Input: part model. Units: mm. Frame: model coordinates. A direction names the side the tool comes from. Round coordinates to 2 decimals unless told otherwise and drop trailing zeros. Loops run counter-clockwise (first coordinate to the right, second up) from the corner with the lowest first, then second, coordinate; pieces in that order, holes last.
(1) Line query: line 1 (Y direction, x = 10.5, z = -10.5); line 2 (Z direction, x = 7.5, y = 22); line 3 (Z direction, x = 9.75, y = 4.5). Output: solid intervals per line, ascending.
(2) Cut plane C-C, the plane x = 12.5. Output: boundary loops of the cut face in (y, z), and give its area (3 significant figures).
(3) Access query for faces 4 (the face through (15, 10, 0)), 5 (the face through (12, 2.8, 12)), 6 (the face through (0, 28, 13.5)), 7 (the face through (-3, 14, 13.5)). Directions: +Z, -Z, +X, -X, +Y, -Y. A direction counts if a zero-diameter tool reaches every point of the face in a straight line with its end or side. Return the directions, or none.
(4) Cut plane D-D, the plane y = 21.5. Output: boundary loops of the cut face in (x, z).
(5) Cut plane B-B, the plane y = 28. Output: boundary loops of the cut face in (x, z), and give its area (3 significant figures).
(6) Cut plane A-A, the plane z = -12.5. Output: boundary loops of the cut face in (x, y), and give its area (3 significant figures).
(7) Draft query along X for faces 1 (the face through (16.5, 5, 0)), 2 (the face through (2, 14, -16.5)), 3 (the face through (-4.496, 10.198, -8.155)). Return one class per face: released by +X, released by -X, zero draft, split by the parting line, or undercut.
(8) First-contact query: pin 1 Ø5 at (y, z) = (16.5, -10) entering from +X; pin 2 Ø5 at (y, z) = (7, 6.5) entering from -X; pin 3 Ø13.5 at (x, z) = (5.5, -2.5) entering from +Y. Flat tips, straight axial feed; report the tip coordinate or a pass-through.
from build123d import *

# Parameters (mm, degrees)
SKETCH1_W                     = 33
SKETCH1_H                     = 33
SKETCH1_W_2                   = 27
SKETCH1_H_2                   = 27
BOSS_EXTRUDE1_DEPTH           = 30
SKETCH3_W                     = 27
SKETCH3_H                     = 30
CUT_EXTRUDE1_DEPTH            = 30
SKETCH4_W                     = 33
SKETCH4_H                     = 1
BOSS_EXTRUDE2_DEPTH           = 33
BOSS_EXTRUDE4_DEPTH           = 4.8
CUT_EXTRUDE3_DEPTH            = 2.8
BOSS_EXTRUDE5_DEPTH           = 4.8
CUT_EXTRUDE5_DEPTH            = 2.8
SKETCH12_W                    = 3
SKETCH12_H                    = 27
CUT_EXTRUDE6_DEPTH            = 10
SKETCH13_W                    = 3
SKETCH13_H                    = 37.394696754
CUT_EXTRUDE7_DEPTH            = 39.800773188
SKETCH15_R                    = 4.5
BOSS_EXTRUDE6_DEPTH           = 33
BOSS_EXTRUDE8_DEPTH           = 27
SKETCH24_R                    = 4.5
BOSS_EXTRUDE7_DEPTH           = 5
BOSS_EXTRUDE7_OTHER_WAY_DEPTH = 16
BOSS_EXTRUDE7_OTHER_WAY_TAPER = -3
SKETCH27_R                    = 4.5
CUT_EXTRUDE12_DEPTH           = 21
CUT_EXTRUDE12_DRAFT           = -5
SKETCH31_R                    = 3
CUT_EXTRUDE14_DEPTH           = 33
CUT_EXTRUDE15_DEPTH           = 20


with BuildPart() as part:
    # Sketch1 → Boss-Extrude1 (new body)
    with BuildSketch(Plane(origin=(0, 0, 0), x_dir=(1, 0, 0), z_dir=(0, 1, 0))):
        Rectangle(SKETCH1_W, SKETCH1_H)
        Rectangle(SKETCH1_W_2, SKETCH1_H_2, mode=Mode.SUBTRACT)
    extrude(amount=BOSS_EXTRUDE1_DEPTH)

    # Sketch3 → Cut-Extrude1 (cut)
    with BuildSketch(Plane(origin=(-13.5, 0, 0), x_dir=(0, 0, -1), z_dir=(1, 0, 0))):
        with Locations((0, 15)):
            Rectangle(SKETCH3_W, SKETCH3_H)
    extrude(amount=-CUT_EXTRUDE1_DEPTH, mode=Mode.SUBTRACT)

    # Sketch4 → Boss-Extrude2 (add)
    with BuildSketch(Plane(origin=(16.5, 0, 0), x_dir=(0, 0, -1), z_dir=(1, 0, 0))):
        with Locations((0, -0.5)):
            Rectangle(SKETCH4_W, SKETCH4_H)
    extrude(amount=-BOSS_EXTRUDE2_DEPTH)

    # Sketch7 → Boss-Extrude4 (add)
    with BuildSketch(Plane(origin=(0, 0, 0), x_dir=(1, 0, 0), z_dir=(0, 1, 0))):
        Polygon((13.5, 13.5), (9.5, 13.5), (13.5, 9.5), align=None)
    extrude(amount=BOSS_EXTRUDE4_DEPTH)

    # Sketch8 → Cut-Extrude3 (cut)
    with BuildSketch(Plane(origin=(0, 0, 0), x_dir=(1, 0, 0), z_dir=(0, 1, 0))):
        Polygon((13.5, 9.5), (9.5, 13.5), (13.5, 13.5), align=None)
    extrude(amount=CUT_EXTRUDE3_DEPTH, mode=Mode.SUBTRACT)

    # Sketch9 → Boss-Extrude5 (add)
    with BuildSketch(Plane(origin=(0, 0, 0), x_dir=(1, 0, 0), z_dir=(0, 1, 0))):
        Polygon((13.5, -13.5), (13.5, -9.5), (9.5, -13.5), align=None)
    extrude(amount=BOSS_EXTRUDE5_DEPTH)

    # Sketch10 → Cut-Extrude5 (cut)
    with BuildSketch(Plane(origin=(0, 0, 0), x_dir=(1, 0, 0), z_dir=(0, 1, 0))):
        Polygon((9.5, -13.5), (13.5, -9.5), (13.5, -13.5), align=None)
    extrude(amount=CUT_EXTRUDE5_DEPTH, mode=Mode.SUBTRACT)

    # Sketch12 → Cut-Extrude6 (cut)
    with BuildSketch(Plane(origin=(0, 0, 0), x_dir=(1, 0, 0), z_dir=(0, 1, 0))):
        with Locations((-15, 0)):
            Rectangle(SKETCH12_W, SKETCH12_H)
    extrude(amount=-CUT_EXTRUDE6_DEPTH, mode=Mode.SUBTRACT)

    # Sketch13 → Cut-Extrude7 (cut, through all)
    with BuildSketch(Plane.XZ.offset(1)):
        with Locations((-15, -2.197348377)):
            Rectangle(SKETCH13_W, SKETCH13_H)
    extrude(amount=-CUT_EXTRUDE7_DEPTH, mode=Mode.SUBTRACT)

    # Sketch15 → Boss-Extrude6 (add, through all)
    with BuildSketch(Plane.XY.offset(16.5)):
        with Locations((0, 10)):
            Circle(SKETCH15_R)
    extrude(amount=-BOSS_EXTRUDE6_DEPTH)

    # Sketch26 → Boss-Extrude8 (add, through all)
    with BuildSketch(Plane.ZY.offset(-13.5)):
        Polygon((13.5, 26), (-13.5, 26), (-13.5, 24), (0, 24), (13.5, 24), align=None)
    extrude(amount=BOSS_EXTRUDE8_DEPTH)

    # Sketch24 → Boss-Extrude7 (add)
    with BuildSketch(Plane(origin=(0, 10, 0), x_dir=(1, 0, 0), z_dir=(0, 1, 0))):
        with Locations(Location((0, 0, 0), (0, 0, 270))):
            Circle(SKETCH24_R)
    extrude(amount=-BOSS_EXTRUDE7_DEPTH)

    # Sketch24 → Boss-Extrude7 other way (add)
    with BuildSketch(Plane(origin=(0, 10, 0), x_dir=(1, 0, 0), z_dir=(0, 1, 0))):
        with Locations(Location((0, 0, 0), (0, 0, 270))):
            Circle(SKETCH24_R)
    extrude(amount=BOSS_EXTRUDE7_OTHER_WAY_DEPTH, taper=BOSS_EXTRUDE7_OTHER_WAY_TAPER)


with BuildPart() as cut_extrude12_tool:
    # Sketch27 → Cut-Extrude12 (with draft: the straight prism first)
    with BuildSketch(Plane(origin=(0, 26, 0), x_dir=(1, 0, 0), z_dir=(0, 1, 0))):
        with Locations(Location((0, 0, 0), (0, 0, 270))):
            Circle(SKETCH27_R)
    extrude(amount=-CUT_EXTRUDE12_DEPTH)
    # Cut-Extrude12: the draft: its side faces are tilted about the plane it starts from
    cut_extrude12_sides = [cut_extrude12_tool.faces().sort_by_distance(p)[0] for p in [
        (0, 15.5, -4.5),
    ]]
    draft(cut_extrude12_sides, Plane(origin=(0, 26, 0), x_dir=(1, 0, 0), z_dir=(0, 1, 0)), CUT_EXTRUDE12_DRAFT)


with BuildPart() as part_1:
    add(part.part)

    # Cut-Extrude12: cut by cut_extrude12_tool
    add(cut_extrude12_tool.part, mode=Mode.SUBTRACT)

    # Sketch31 → Cut-Extrude14 (cut)
    with BuildSketch(Plane.XY.offset(16.5)):
        with Locations((-0.171414506, 10)):
            Circle(SKETCH31_R)
    extrude(amount=-CUT_EXTRUDE14_DEPTH, mode=Mode.SUBTRACT)

    # Sketch32 → Cut-Extrude15 (cut)
    with BuildSketch(Plane(origin=(0, 30, 0), x_dir=(1, 0, 0), z_dir=(0, 1, 0))):
        Polygon((13.5, 13.5), (13.5, 17.645785923), (20.004532671, 17.645785923), (20.004532671, -18.642828809), (13.5, -18.642828809), (13.5, -13.5), align=None)
    extrude(amount=-CUT_EXTRUDE15_DEPTH, mode=Mode.SUBTRACT)


solid = part_1.part
Reported:
1. line 1: y = -1 to 0, 24 to 26
1. line 2: z = -16.5 to -13.5, 13.5 to 16.5
1. line 3: z = -16.5 to -13.25, 13.25 to 16.5
2. outline: (-1, -16.5) - (30, -16.5) - (30, -13.5) - (26, -13.5) - (26, 13.5) - (30, 13.5) - (30, 16.5) - (-1, 16.5) - close; hole (0, -13.5) - (2.8, -13.5) - (2.8, -10.5) - (4.8, -10.5) - (4.8, -13.5) - (24, -13.5) - (24, 13.5) - (4.8, 13.5) - (4.8, 10.5) - (2.8, 10.5) - (2.8, 13.5) - (0, 13.5) - close
2. area: 279 mm2
3. face 4: +Z, -Z, +X, +Y
3. face 5: -X
3. face 6: +X, -X, +Y
3. face 7: none
4. outline: (-13.5, -16.5) - (13.5, -16.5) - (13.5, -13.5) - (-13.5, -13.5) - close; (-13.5, 13.5) - (13.5, 13.5) - (13.5, 16.5) - (-13.5, 16.5) - close; circle Ø10.21 at (0, 0); hole circle Ø8.21 at (0, 0)
5. outline: (-13.5, -16.5) - (13.5, -16.5) - (13.5, -13.5) - (-13.5, -13.5) - close; (-13.5, 13.5) - (13.5, 13.5) - (13.5, 16.5) - (-13.5, 16.5) - close
5. area: 162 mm2
6. outline: (-13.5, -1) - (16.5, -1) - (16.5, 10) - (13.5, 10) - (13.5, 4.8) - (10.5, 4.8) - (10.5, 2.8) - (13.5, 2.8) - (13.5, 0) - (-13.5, 0) - close; (-13.5, 24) - (13.5, 24) - (13.5, 26) - (-13.5, 26) - close; circle Ø9 at (0, 10); hole circle Ø6 at (-0.17, 10)
6. area: 155 mm2
7. face 1: released by +X
7. face 2: zero draft
7. face 3: undercut
8. pin 1: stops at x = 2.06
8. pin 2: stops at x = -4.47
8. pin 3: stops at y = 26
